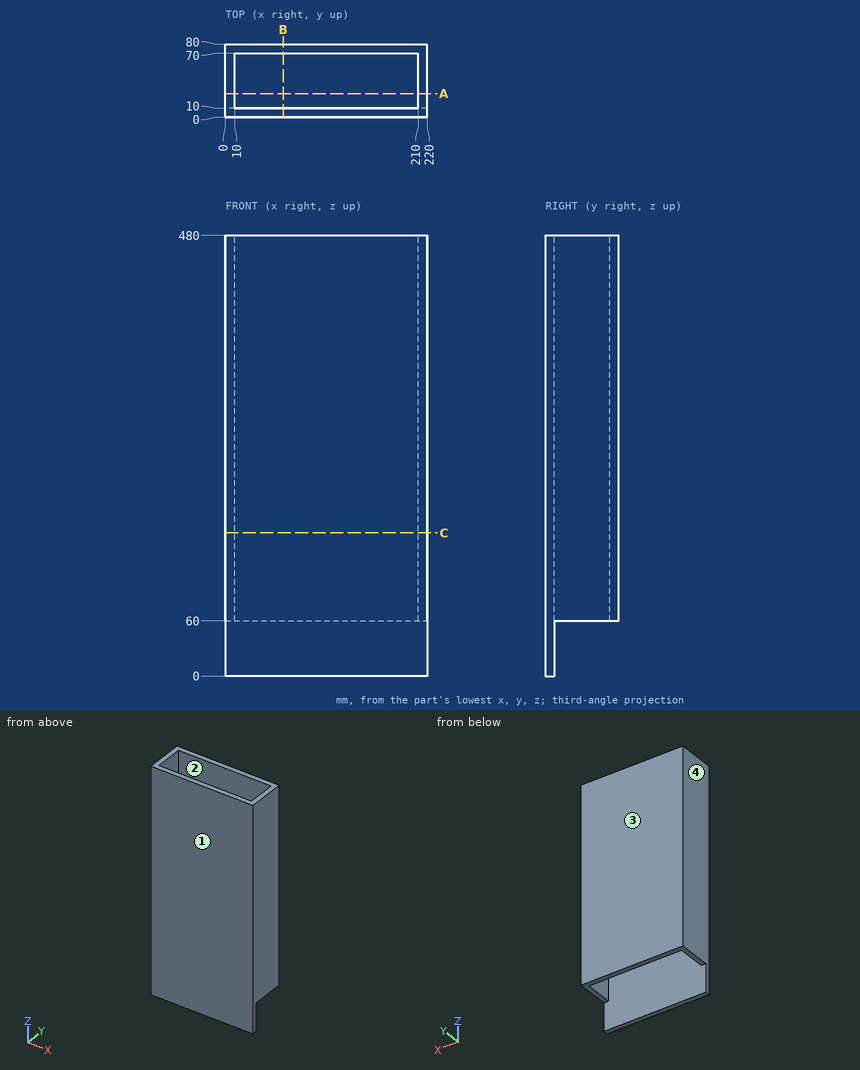
For this review, use the dimensioned drawing (mm, ordinates from the lowest corner) and the shaded views. Coordinates: 2 decimals unless noted, no trailing zeros. Loops run counter-clockwise (first coordinate to the right, second up) from the corner with the lowest first, then second, coordinate; pieces in that order, holes last. Notation, with made-up numbers: (-3.75, 19) -> (25.25, 19) arc R20 ccw to (25.25, 50) -> close; hole circle Ø11 at (8.5, 15). An arc over 180 degrees is marked (long way). Use a Markdown table: item, result. Add a question column.
1. Add section A-A on y = 26. Write out the cut boundary in (x, z).
2. Draft analysis for pull direction Y (two halves, no side actions). For the marked faces 1, 2, 3 and 4, state which applies: pulls with the +Y half, pulls with the -Y half, needs draft (parallel to the pull), parting line crosses it, or undercut.
3. Clearance check with a flat-ended pin moving along its axis: pin 1 Ø10 at (x, y) = (23, 68.5) entering from -Z. State where the tip first meets the part, or that it passes through.
4. To check wall thickness, follow line 1 (Y direction, x = 93, z = 169); line 2 (X direction, y = 52, z = 245.5); line 3 (Y direction, x = 18, z = 56.5). State the ranges of each line that lie inside material, in increasing order.
5. Add section B-B on x = 63. Write out the cut boundary in (y, z).
6. Add section C-C on z = 156. Write out the cut boundary in (x, y).
Returned:
| question | item | result |
|---|---|---|
| 1 | outline | (0, 60) -> (10, 60) -> (10, 480) -> (0, 480) -> close; (210, 60) -> (220, 60) -> (220, 480) -> (210, 480) -> close |
| 2 | face 1 | pulls with the -Y half |
| 2 | face 2 | undercut |
| 2 | face 3 | pulls with the +Y half |
| 2 | face 4 | needs draft |
| 3 | pin 1 | stops at z = 60 |
| 4 | line 1 | y = 0 to 10, 70 to 80 |
| 4 | line 2 | x = 0 to 10, 210 to 220 |
| 4 | line 3 | y = 0 to 10 |
| 5 | outline | (0, 0) -> (10, 0) -> (10, 480) -> (0, 480) -> close; (70, 60) -> (80, 60) -> (80, 480) -> (70, 480) -> close |
| 6 | outline | (0, 0) -> (220, 0) -> (220, 80) -> (0, 80) -> close; hole (10, 10) -> (210, 10) -> (210, 70) -> (10, 70) -> close |
